Autodesk Inventor part; units mm, degrees
ref_plane "YZ Plane" through (0, 0, 0) normal (1, 0, 0) x (0, 1, 0)
ref_plane "XZ Plane" through (0, 0, 0) normal (0, 1, 0) x (-1, 0, 0)
ref_plane "XY Plane" through (0, 0, 0) normal (0, 0, 1) x (1, 0, 0)
sketch "Sketch1" plane through (0, 0, 0) normal (0, 1, 0) x (-1, 0, 0)
  circle A0 centre (0, 0) radius 8.5
  dimension "d1" = 17
extrude "Extrusion1" add sketch "Sketch1" along normal blind 9
sketch "Sketch2" plane through (0, 0, 0) normal (0, -1, 0) x (1, 0, 0)
  circle A0 centre (0, 0) radius 6.5
  dimension "d4" = 13
extrude "Extrusion2" cut sketch "Sketch2" against normal blind 5.5
sketch "Sketch4" plane through (0, 0, 0) normal (1, 0, 0) x (0, 1, 0)
  line L0 (9, -8.5) -> (9, 8.5)
  circle A0 centre (9, 0) radius 2.05
  point P0 (0, 0)
  dimension "d7" = 4.1
extrude "Extrusion3" cut sketch "Sketch4" along normal mid plane 8.1
fillet "Fillet1" radius 1.5 1 edges at (8.5, 9, 0)
properties part number "magnet_holder"
The listing builds one solid part. Answer for the finished solid, in the listing's coordinates (mm). A direction names the side the tool comes from. Give positions to 0.01 mm unless a question says otherwise; leave off trailing zeros. Order: outer loops, then holes, each group sorted by start corner. A loop starts at its lowest first (then second) coordinate and runs counter-clockwise, first axis right, second up. Notation, with made-up numbers: (64, -40) -> (104, -40) arc R19 ccw to (104, -3) -> close; hole circle Ø4 at (81.5, 11.5). An arc over 180 degrees is marked (long way). Answer as a JSON object with one key per item and string values. Group by question number.
Item 1: The part is cut by section C-C on y = 8.5. Write down the section's boundary in (x, z), and give its area (3 significant figures).
Item 2: Consider L1, parallel to Z at x = 0, y = 3.55; L2, parallel to X at y = 4.25, z = 2; L3, parallel to X at y = 4.5, z = 4.5. Determine where each line is inside the solid, lowest interval first. Write a range as from..to.
Item 3: The part is cut by section A-A on z = 0. Write down the section's boundary in (x, y).
Item 4: The part is cut by section D-D on y = 5.75. Write down the section's boundary in (x, z), and give its area (3 significant figures).
Item 5: The part is cut by section B-B on x = 0. Write down the section's boundary in (y, z), and give its area (3 significant figures).
Item 6: Determine the mould class of faces 4 (the flat face through (-4.4, 0, -5)), 5 (the flat face through (-4.05, 8, 0)), 6 (the cylindrical face through (-4.57, 3.698, -7.167)) for opening direction X: pulls with the +X half, pulls with the -X half, needs draft (parallel to the pull), parting line crosses it, or undercut.
Item 7: Flat-ended cylindrical pins translate along their axes: pin 1 (4 mm diameter, centred on x = 5, y = 3.5, fed in from -Z); pin 2 (1.6 mm diameter, centred on y = 7.5, z = 0.5, fed in from +X); pin 3 (8 mm diameter, centred on x = 0, z = 0, fed in from -Y); pin 4 (2 mm diameter, centred on y = 4, z = -2.5, fed in from +X). Find the tip coordinate at first contact, or state that the pin passes through.
Item 8: A tool of negligible diameter and unlimited length cuts with its end or side. For faces 1 (the flat face through (4.05, 8, 0)), 2 (the flat face through (0, 9, -3)), 3 (the flat face through (0, 5.5, 0)), from which of +Z, -Z, +X, -X, +Y, -Y can it reach the whole face along a straight path? Write none if from no direction.
Result set:
{
 "1": {"outline": "circle Ø16.24 at (0, 0); hole (-4.05, -1.99) -> (4.05, -1.99) -> (4.05, 1.99) -> (-4.05, 1.99) -> close", "area": "175 mm²"},
 "2": {"L1": "-8.5..-6.5, 6.5..8.5", "L2": "-8.26..-6.18, 6.18..8.26", "L3": "-7.21..-4.69, 4.69..7.21"},
 "3": {"outline": "(-8.5, 0) -> (-6.5, 0) -> (-6.5, 5.5) -> (6.5, 5.5) -> (6.5, 0) -> (8.5, 0) -> (8.5, 7.5) arc R1.5 ccw to (7, 9) -> (4.05, 9) -> (4.05, 6.95) -> (-4.05, 6.95) -> (-4.05, 9) -> (-7, 9) arc R1.5 ccw to (-8.5, 7.5) -> close"},
 "4": {"outline": "circle Ø17 at (0, 0)", "area": "227 mm²"},
 "5": {"outline": "(0, -8.5) -> (7.5, -8.5) arc R1.5 ccw to (9, -7) -> (9, -2.05) arc R2.05 cw to (9, 2.05) -> (9, 7) arc R1.5 ccw to (7.5, 8.5) -> (0, 8.5) -> (0, 6.5) -> (5.5, 6.5) -> (5.5, -6.5) -> (0, -6.5) -> close", "area": "73.9 mm²"},
 "6": {"face 4": "needs draft", "face 5": "undercut", "face 6": "parting line crosses it"},
 "7": {"pin 1": "z = -7.95", "pin 2": "x = 8.5", "pin 3": "y = 5.5", "pin 4": "x = 8.37"},
 "8": {"face 1": "+Y", "face 2": "+Z, -Z, +X, -X, +Y", "face 3": "-Y"}
}
